Build history of the part. All positions in model axes, mm. A direction names the side the tool comes from. Round coordinates to 2 decimals unless told otherwise and drop trailing zeros. Loops run counter-clockwise (first coordinate to the right, second up) from the corner with the lowest first, then second, coordinate; pieces in that order, holes last. Notation, with made-up numbers: (69, 75.25) - (99, 75.25) arc R10 ccw to (99, 87.25) - close; hole circle Ø6 at (-9, 83). An arc over 180 degrees is marked (long way). Put each result on its own line as item: value. Start each with the question number.
Autodesk Fusion 360 part; units mm, degrees
sketch "Sketch1" plane through (0, 0, 0) normal (0, 0, 1) x (1, 0, 0)
  circle A0 centre (0, 0) radius 12.75
  circle A1 centre (0, 9) radius 1.55
  circle A2 centre (-7.7942, -4.5) radius 1.55
  circle A3 centre (7.7942, -4.5) radius 1.55
  dimension "d1" = 25.5
  dimension "d2" = 3.1
  dimension "d3" = 9
  dimension "d5" = 360
extrude "Extrude1" add sketch "Sketch1" along normal blind 4
sketch "Sketch2" plane through (0, 0, 4) normal (0, 0, 1) x (-1, 0, 0)
  circle A0 centre (-7.7942, 4.5) radius 1.55
  circle A1 centre (7.7942, 4.5) radius 1.55
  circle A2 centre (0, -9) radius 1.55
  circle A3 centre (0, 0) radius 12.75
  circle A4 centre (0, 0) radius 6.25
  circle A5 centre (0, 0) radius 4
  dimension "d8" = 12.5
  dimension "d9" = 8
extrude "Extrude2" add sketch "Sketch2" along normal blind 15 contours A4
extrude "Extrude3" cut 1 faces at (-0.9485, -1.8197, 4) along direction (0, 0, -1) blind 7
1) Which spindle directions (+Z, -Z, +X, -X, +Y, -Y) get a long thin tool onto all of the face, cutting with end or side? Do faces 1 (the face through (9.27, -4.97, 1.97)), 2 (the face through (-5.96, 1.88, 11.4)). Say none if no direction does.
2) Pull direction X, two halves, no side cores. Call faces 3 (the face through (3, 3, 0)), 4 (the face through (-2.764, 12.447, 1.972)), 5 (the face through (-0.336, 10.513, 1.972)): pulls with the +X half, pulls with the -X half, needs draft (parallel to the pull), parting line crosses it, or undercut.
3) Slice it at D-D, the plane x = 7. Write the cut outline in (y, z).
4) Drill centre lines: line 1 (Y direction, x = 0, z = 5.75); line 2 (Z direction, x = -6.5, y = 3); line 3 (X direction, y = 2.25, z = 12.75). Where is each one in solid material? Low to high. Write a range as [from, to].
5) Slice it at C-C, the plane y = -4.5. Write the cut outline in (x, z), and give its area (3 significant figures).
6) Slice it at B-B, the plane z = 1.75. Write the cut outline in (x, y), and give its area (3 significant figures).
7) Drop flat-ended pins along their axis: pin 1 Ø1.5 at (x, y) = (6, 8) entering from +Z; pin 2 Ø2.5 at (x, y) = (-7.79, -4.5) entering from -Z; pin 3 Ø4 at (x, y) = (7.79, -4.5) entering from -Z; pin 4 Ø2 at (x, z) = (6.5, 9) entering from -Y. Give the stop position or say it passes through.
8) Slice it at A-A, the plane x = 0. Write the cut outline in (y, z), and give its area (3 significant figures).
Taken from the geometry:
1. face 1: +Z, -Z
1. face 2: +Z
2. face 3: needs draft
2. face 4: parting line crosses it
2. face 5: undercut
3. outline: (-10.66, 0) - (-5.83, 0) - (-5.83, 4) - (-10.66, 4) - close; (-3.17, 0) - (10.66, 0) - (10.66, 4) - (-3.17, 4) - close
4. line 1: y = [-6.25, -4], [4, 6.25]
4. line 2: z = [0, 4]
4. line 3: x = [-5.83, -3.31], [3.31, 5.83]
5. outline: (-11.93, 0) - (-9.34, 0) - (-9.34, 4) - (-11.93, 4) - close; (-6.24, 0) - (6.24, 0) - (6.24, 4) - (4.34, 4) - (4.34, 19) - (-4.34, 19) - (-4.34, 4) - (-6.24, 4) - close; (9.34, 0) - (11.93, 0) - (11.93, 4) - (9.34, 4) - close
5. area: 201 mm2
6. outline: circle Ø25.5 at (0, 0); hole circle Ø3.1 at (-7.79, -4.5); hole circle Ø8 at (0, 0); hole circle Ø3.1 at (0, 9); hole circle Ø3.1 at (7.79, -4.5)
6. area: 438 mm2
7. pin 1: stops at z = 4
7. pin 2: passes through
7. pin 3: stops at z = 0
7. pin 4: stops at y = -2.97
8. outline: (-12.75, 0) - (-4, 0) - (-4, 19) - (-6.25, 19) - (-6.25, 4) - (-12.75, 4) - close; (4, 0) - (7.45, 0) - (7.45, 4) - (6.25, 4) - (6.25, 19) - (4, 19) - close; (10.55, 0) - (12.75, 0) - (12.75, 4) - (10.55, 4) - close
8. area: 125 mm2
